from build123d import *

# Parameters (mm, degrees)
F0_W     = 319.505253
F0_H     = 37.063959
F1_DEPTH = 76.2
F2_W     = 55.612809
F2_H     = 19.239029
F2_W_2   = 55.61281
F2_H_2   = 18.938417
F3_DEPTH = 129.54
F4_W     = 69.768153
F4_H     = 27.621901
F4_W_2   = 78.345757
F4_H_2   = 29.128553
F5_DEPTH = 104.14


with BuildPart() as f1:
    # F0 (on Front) → F1 (new body)
    with BuildSketch(Plane.XZ):
        with Locations((33.688419, -34.904941)):
            Rectangle(F0_W, F0_H)
    extrude(amount=F1_DEPTH)

    # F2 (on face) → F3 (join)
    with BuildSketch(Plane.XY.offset(-16.372962)):
        with Locations((-35.000917, -37.726529)):
            Rectangle(F2_W, F2_H)
        with Locations((98.169219, -36.073173)):
            Rectangle(F2_W_2, F2_H_2)
    extrude(amount=F3_DEPTH)

    # F4 (on face) → F5 (join)
    with BuildSketch(Plane.XY.offset(113.167038)):
        with Locations((-34.884076, -37.289564)):
            Rectangle(F4_W, F4_H)
        with Locations((99.47876, -36.787349)):
            Rectangle(F4_W_2, F4_H_2)
    extrude(amount=F5_DEPTH)


solid = f1.part
Source: CAD feature listing. Evaluate the final solid. Frame: model axes, mm. A direction names the side the tool comes from. Give positions to 0.01 mm unless a question says otherwise; leave off trailing zeros. Order: outer loops, then holes, each group sorted by start corner. A loop starts at its lowest first (then second) coordinate and runs counter-clockwise, first axis right, second up. Notation, with made-up numbers: (57, 15.25) -> (93, 15.25) arc R24 cw to (93, 40.25) -> close; hole circle Ø8 at (28, 63). An arc over 180 degrees is marked (long way). Write item = value, one per line.
Item 1: Section query C-C (x = 108). Output: boundary loops of the cut face in (y, z).
Check result:
outline = (-76.2, -53.44) -> (0, -53.44) -> (0, -16.37) -> (-26.6, -16.37) -> (-26.6, 113.17) -> (-22.22, 113.17) -> (-22.22, 217.31) -> (-51.35, 217.31) -> (-51.35, 113.17) -> (-45.54, 113.17) -> (-45.54, -16.37) -> (-76.2, -16.37) -> close
Item 2: Section query A-A (y = -39.5). Output: boundary loops of the cut face in (x, z), then the cut area to 3 significant figures.
Check result:
outline = (-126.06, -53.44) -> (193.44, -53.44) -> (193.44, -16.37) -> (125.98, -16.37) -> (125.98, 113.17) -> (138.65, 113.17) -> (138.65, 217.31) -> (60.31, 217.31) -> (60.31, 113.17) -> (70.36, 113.17) -> (70.36, -16.37) -> (-7.19, -16.37) -> (-7.19, 113.17) -> (0, 113.17) -> (0, 217.31) -> (-69.77, 217.31) -> (-69.77, 113.17) -> (-62.81, 113.17) -> (-62.81, -16.37) -> (-126.06, -16.37) -> close
area = 41,700 mm²
Item 3: Mould query, pull axis X, two halves, no side actions, for faces 1 (the face through (98, -26.604, 47)), 2 (the face through (125.976, -36, 47)), 3 (the face through (60.306, -37, 165)). Classes: +X half, -X half, draft (parallel to the pull), parting line (faces both ways), or undercut.
Check result:
face_1 = draft
face_2 = +X half
face_3 = undercut
Item 4: Set-up query: faces 4 (the face through (-35, -47.346, 47)), 5 (the face through (138.652, -37, 165)), 6 (the face through (99, -46, 113.167)), 7 (the face through (98, -45.542, 47)), 8 (the face through (99, -22.223, 165)). Return all of +Z, -Z, +X, -X, +Y, -Y with unobstructed straight access to the full face (end or side cutting, diameter ignored); none if empty.
Check result:
face_4 = +X, -X, -Y
face_5 = +Z, +X, +Y, -Y
face_6 = none
face_7 = +X, -Y
face_8 = +Z, +X, -X, +Y
Item 5: Section query D-D (z = 46.5). Output: boundary loops of the cut face in (x, y).
Check result:
outline = (-62.81, -47.35) -> (-7.19, -47.35) -> (-7.19, -28.11) -> (-62.81, -28.11) -> close; (70.36, -45.54) -> (125.98, -45.54) -> (125.98, -26.6) -> (70.36, -26.6) -> close
Item 6: Contact query for flat-ended pins moving along their axis: pin 1 (2 mm diameter, centred on y = -37.5, z = 15.5, fed in from -X); pin 2 (8 mm diameter, centred on y = -22.5, z = 127.5, fed in from -X); pin 3 (6 mm diameter, centred on y = -35, z = 72.5, fed in from +X). Output: stop coordinate, or through.
Check result:
pin_1 = -62.81
pin_2 = -69.77
pin_3 = 125.98
Item 7: Ray query, probe 1 along X at (y, z) = (-42, 126.5); probe 2 along Z at (x, y) = (127.5, -40); probe 3 along Z at (x, y) = (42.5, -14). Return the intervals inside material, ascending.
Check result:
probe_1 = -69.77 to 0, 60.31 to 138.65
probe_2 = -53.44 to -16.37, 113.17 to 217.31
probe_3 = -53.44 to -16.37
Item 8: Section query B-B (z = 142.5). Output: boundary loops of the cut face in (x, y).
Check result:
outline = (-69.77, -51.1) -> (0, -51.1) -> (0, -23.48) -> (-69.77, -23.48) -> close; (60.31, -51.35) -> (138.65, -51.35) -> (138.65, -22.22) -> (60.31, -22.22) -> close
